Part model, mm, in its own coordinate system. Coordinates: 2 decimals unless noted, no trailing zeros. Loops run counter-clockwise (first coordinate to the right, second up) from the corner with the lowest first, then second, coordinate; pieces in that order, holes last. Notation, with made-up numbers: (54.25, -35) - (111.25, -35) arc R21 cw to (111.25, -28) - close; hole circle Ø4 at (-34, 67.5). An arc over 180 degrees is marked (long way). Use a Markdown table: item, result. Add a question column.
1. Band-saw the part on D-D, the plane z = 83.5. Give the cut face in (x, y).
2. Wall check: probe 1 along Z at (x, y) = (-6.5, -13.75); probe 2 along X at (y, z) = (-12, -17.5); probe 3 along X at (y, z) = (-9.25, 2). Give the ranges that are in metal, low to high. Write a range as [from, to].
3. Drop flat-ended pins along their axis: pin 1 (6 mm diameter, centred on x = -35.5, y = -4.5, fed in from -Z); pin 2 (1 mm diameter, centred on y = -23, z = 5, fed in from +X); pin 3 (4 mm diameter, centred on x = -90, y = -19.5, fed in from +Z); pin 4 (10.5 mm diameter, centred on x = -2.6, z = 40.5, fed in from +Y). Give the stop position or say it passes through.
4. Band-saw the part on C-C, the plane x = -51. Give the cut face in (y, z), plus the area to 3 significant figures.
5. Pull direction Z, two halves, no side cores. Call faces 1 (the flat face through (-63, 0, 38)), 2 (the cylindrical face through (-77.08, -12.52, -31.33)), 3 (the cylindrical face through (-41.808, -12.878, 92.519)): pulls with the +Z half, pulls with the -Z half, needs draft (parallel to the pull), parting line crosses it, or undercut.
6. Band-saw the part on A-A, the plane x = -122. Give the cut face in (y, z), plus the area to 3 significant figures.
7. Band-saw the part on B-B, the plane y = -15. Count the separate pieces of the cut face and the enclosed holes in it, plus the area to 3 significant figures.
from build123d import *

# Parameters (mm, degrees)
F0_R            = 69.6849
F1_DEPTH        = 25.4
F2_R            = 5.7253497259
F3_DEPTH        = 25.401
F3_COPIES_COUNT = 10


# Not quite as in the source:
# - a pattern or mirror of a feature is missing from the dataset's text; its kind, count and spacing are read off the source's solid


with BuildPart() as f1:
    # F0 (on Front) → F1 (new body)
    with BuildSketch(Plane.XZ):
        with Locations((-61.9692653418, 36.6955287755)):
            Circle(F0_R)
    extrude(amount=F1_DEPTH)

    # F2 (on face) → F3 (cut, through all)
    with BuildSketch(Plane.XZ.offset(25.4)):
        with Locations((-83.9317291975, 91.9884815812)):
            Circle(F2_R)
    f3 = extrude(amount=-F3_DEPTH, mode=Mode.SUBTRACT)

    # F3_copies: F3 ×10 about axis
    f3_copies_axis = Axis((-61.969265, 0, 36.695529), (0, 1, 0))
    for i in range(1, F3_COPIES_COUNT):
        add(f3.rotate(f3_copies_axis, i * 360 / F3_COPIES_COUNT), mode=Mode.SUBTRACT)


solid = f1.part
Geometry check:
| question | item | result |
|---|---|---|
| 1 | outline | (-113.6, -25.4) - (-10.34, -25.4) - (-10.34, 0) - (-113.6, 0) - close |
| 2 | probe 1 | z = [-5.48, 2.48], [7.27, 36.31], [44.68, 78.88] |
| 2 | probe 2 | x = [-105.77, -81.27], [-72.13, -45.63], [-34.39, -18.16] |
| 2 | probe 3 | x = [-122.4, -112.46], [-103.08, -16.65], [-6.75, -1.54] |
| 3 | pin 1 | stops at z = -28.92 |
| 3 | pin 2 | stops at x = 0.34 |
| 3 | pin 3 | stops at z = 101.34 |
| 3 | pin 4 | passes through |
| 4 | outline | (-25.4, -32.12) - (0, -32.12) - (0, 90.02) - (-25.4, 90.02) - close; (-25.4, 98.65) - (0, 98.65) - (0, 105.51) - (-25.4, 105.51) - close |
| 4 | area | 3,280 mm^2 |
| 5 | face 1 | needs draft |
| 5 | face 2 | parting line crosses it |
| 5 | face 3 | undercut |
| 6 | outline | (-25.4, 1.31) - (0, 1.31) - (0, 27.21) - (-25.4, 27.21) - close; (-25.4, 38.58) - (0, 38.58) - (0, 72.08) - (-25.4, 72.08) - close |
| 6 | area | 1,510 mm^2 |
| 7 | separate pieces | 1 |
| 7 | enclosed holes | 10 |
| 7 | area | 14,200 mm^2 |
